Geometry check sheet. Reference: the model listing, model coordinates, mm. A direction names the side the tool comes from. Coordinates: 2 decimals unless noted, no trailing zeros. Order: outer loops, then holes, each group sorted by start corner. A loop starts at its lowest first (then second) coordinate and runs counter-clockwise, first axis right, second up. Notation, with made-up numbers: M 11.25,49.5 L 31.25,49.5 A20 cw 31.25,80.5 Z; hole C -34.75,44 d3. An arc over 180 degrees is marked long. Use CSV: the item, a comma, the result in double quotes. Start each with the question number.
```python
from build123d import *

# Parameters (mm, degrees)
SKETCH_2_W          = 170
SKETCH_2_H          = 20
EXTRUDE_1_DEPTH     = 23
CUT_EXTRUDE_1_DEPTH = 173.710740836
SKETCH_4_W          = 17
SKETCH_4_H          = 13
CUT_EXTRUDE_2_DEPTH = 30
CUT_EXTRUDE_3_DEPTH = 173.710740836
SKETCH_6_W          = 17.5
SKETCH_6_H          = 14.5
CUT_EXTRUDE_4_DEPTH = 173.710740836
SKETCH_7_W          = 27
SKETCH_7_H          = 23
SKETCH_7_R          = 1.25
EXTRUDE_2_DEPTH     = 3
CUT_EXTRUDE_START   = -3
SKETCH_7_3_R        = 2
CUT_EXTRUDE_5_DEPTH = 1.5


with BuildPart() as part:
    # 草图2 → 凸台-拉伸1 (new body)
    with BuildSketch(Plane(origin=(0, 0, 0), x_dir=(1, 0, 0), z_dir=(0, 1, 0))):
        with Locations((85, -10)):
            Rectangle(SKETCH_2_W, SKETCH_2_H)
    extrude(amount=EXTRUDE_1_DEPTH)

    # 草图3 → 切除-拉伸1 (cut, through all)
    with BuildSketch(Plane(origin=(0, 23, 0), x_dir=(1, 0, 0), z_dir=(0, 1, 0))):
        with BuildLine():
            ThreePointArc((161.6, -10), (159.341699476, -8.541699476), (158.941699476, -11.2))
            Line((158.941699476, -11.2), (161.058300524, -11.2))
            ThreePointArc((161.058300524, -11.2), (161.458300524, -10.658300524), (161.6, -10))
        make_face()
        with BuildLine():
            ThreePointArc((126.6, -10), (124.341699476, -8.541699476), (123.941699476, -11.2))
            Line((123.941699476, -11.2), (126.058300524, -11.2))
            ThreePointArc((126.058300524, -11.2), (126.458300524, -10.658300524), (126.6, -10))
        make_face()
    extrude(amount=-CUT_EXTRUDE_1_DEPTH, mode=Mode.SUBTRACT)

    # 草图4 → 切除-拉伸2 (cut)
    with BuildSketch(Plane(origin=(170, 0, 0), x_dir=(0, 0, -1), z_dir=(1, 0, 0))):
        with Locations((-8.5, 11.5)):
            Rectangle(SKETCH_4_W, SKETCH_4_H)
    extrude(amount=-CUT_EXTRUDE_2_DEPTH, mode=Mode.SUBTRACT)

    # 草图5 → 切除-拉伸3 (cut, through all)
    with BuildSketch(Plane(origin=(0, 23, 0), x_dir=(1, 0, 0), z_dir=(0, 1, 0))):
        with BuildLine():
            Line((117.5, -17), (117.5, -10))
            ThreePointArc((117.5, -10), (125, -2.5), (132.5, -10))
            Line((132.5, -10), (132.5, -17))
            Line((132.5, -17), (152.5, -17))
            Line((152.5, -17), (152.5, -10))
            ThreePointArc((152.5, -10), (160, -2.5), (167.5, -10))
            Line((167.5, -10), (167.5, -17))
            Line((167.5, -17), (170, -17))
            Line((170, -17), (170, 0))
            Line((170, 0), (0, 0))
            Line((0, 0), (0, -20))
            Line((0, -20), (102.5, -20))
            Line((102.5, -20), (102.5, -17))
            Line((102.5, -17), (117.5, -17))
        make_face()
    extrude(amount=-CUT_EXTRUDE_3_DEPTH, mode=Mode.SUBTRACT)

    # 草图6 → 切除-拉伸4 (cut, through all)
    with BuildSketch(Plane(origin=(0, 23, 0), x_dir=(1, 0, 0), z_dir=(0, 1, 0))):
        Polygon((152.5, -17), (102.5, -17), (102.5, -20), (170, -20), (170, -17), align=None)
        with Locations((161.25, -9.75)):
            Rectangle(SKETCH_6_W, SKETCH_6_H)
    extrude(amount=-CUT_EXTRUDE_4_DEPTH, mode=Mode.SUBTRACT)

    # 草图7 → 凸台-拉伸2 (add)
    with BuildSketch(Plane.XY.offset(17)):
        with Locations((125, 11.5)):
            Rectangle(SKETCH_7_W, SKETCH_7_H)
        with Locations((114.5, 19)):
            Circle(SKETCH_7_R, mode=Mode.SUBTRACT)
        with Locations((114.5, 4)):
            Circle(SKETCH_7_R, mode=Mode.SUBTRACT)
        with Locations((135.5, 4)):
            Circle(SKETCH_7_R, mode=Mode.SUBTRACT)
        with Locations((135.5, 19)):
            Circle(SKETCH_7_R, mode=Mode.SUBTRACT)
    extrude(amount=-EXTRUDE_2_DEPTH)

    # 草图7<3> → 切除-拉伸5 (cut)
    with BuildSketch(Plane.XY.offset(17).offset(CUT_EXTRUDE_START)):
        with Locations(Location((114.5, 19, 0), (0, 0, 180))):
            Circle(SKETCH_7_3_R)
        with Locations(Location((114.5, 4, 0), (0, 0, 180))):
            Circle(SKETCH_7_3_R)
        with Locations(Location((135.5, 4, 0), (0, 0, 180))):
            Circle(SKETCH_7_3_R)
        with Locations(Location((135.5, 19, 0), (0, 0, 180))):
            Circle(SKETCH_7_3_R)
    extrude(amount=CUT_EXTRUDE_5_DEPTH, mode=Mode.SUBTRACT)


solid = part.part
```
1) Gauge pin test, flat ends, axial feed: P1, Ø4, axis at y = 2.5, z = 10.5, coming from the +X side; P2, Ø3, axis at y = 17, z = 7, coming from the +X side; P3, Ø1.2, axis at y = 11, z = 12, coming from the -X side. Record the tip position at first contact, or that the pin passes through.
2) Section check A-A on x = 135.5. Record the boundary of the cut face in (y, z), then the cut area to 3 significant figures.
3) Set-up check for faces 5 (the face through (125, 12, 17)), 6 (the face through (113, 4, 15.5)), 7 (the face through (135, 12, 14)), 8 (the face through (125, 12, 11.2)), 9 (the face through (124.8, 0, 11.5)): record each of +Z, -Z, +X, -X, +Y, -Y from which the full face is reachable in a straight line by a thin tool's end or side.
4) Material ranges on line 1 along X through (y, z) = (19, 14.45); line 2 along Y through (x, z) = (114.5, 14.6); line 3 along X through (y, z) = (8.5, 10), recorded low to high.
5) Section check D-D on z = 10.5. Record the boundary of the cut face in (x, y).
6) Draft check along Y on faces 1 (the face through (117.5, 12, 12)), 2 (the face through (115.655, 3.521, 16.26)), 3 (the face through (116.498, 18.912, 14.74)), 4 (the face through (124.8, 23, 11.5)). Enter one of: +Y half, -Y half, draft (parallel to the pull), parting line (faces both ways), or undercut.
7) Section check B-B on y = 19. Record the boundary of the cut face in (x, z), then the cut area to 3 significant figures.
8) Section check C-C on x = 125. Record the boundary of the cut face in (y, z).
Results are:
1,P1,"stops at x = 132.5"
1,P2,"stops at x = 132.35"
1,P3,"stops at x = 117.5"
2,outline,"M 0,14 L 2,14 L 2,15.5 L 2.75,15.5 L 2.75,17 L 0,17 Z; M 5.25,15.5 L 6,15.5 L 6,14 L 17,14 L 17,15.5 L 17.75,15.5 L 17.75,17 L 5.25,17 Z; M 20.25,15.5 L 21,15.5 L 21,14 L 23,14 L 23,17 L 20.25,17 Z"
2,area,"49.5 mm²"
3,face 5,"+Z, +X, -X, +Y, -Y"
3,face 6,"-Z"
3,face 7,"-Z, +X, +Y, -Y"
3,face 8,"+Y, -Y"
3,face 9,"+Z, -Z, +X, -X, -Y"
4,line 1,"x = 111.5 to 112.5, 116.5 to 133.5, 137.5 to 138.5"
4,line 2,"y = 0 to 2, 6 to 17, 21 to 23"
4,line 3,"x = 117.5 to 123.4, 126.6 to 132.5"
5,outline,"M 117.5,0 L 123.48,0 L 123.48,23 L 117.5,23 Z; M 126.52,0 L 132.5,0 L 132.5,23 L 126.52,23 Z"
6,face 1,"draft"
6,face 2,"undercut"
6,face 3,"undercut"
6,face 4,"+Y half"
7,outline,"M 111.5,14 L 112.5,14 L 112.5,15.5 L 113.25,15.5 L 113.25,17 L 111.5,17 Z; M 115.75,15.5 L 116.5,15.5 L 116.5,14 L 117.5,14 L 117.5,10 A7.5 ccw 132.5,10 L 132.5,14 L 133.5,14 L 133.5,15.5 L 134.25,15.5 L 134.25,17 L 115.75,17 Z; M 136.75,15.5 L 137.5,15.5 L 137.5,14 L 138.5,14 L 138.5,17 L 136.75,17 Z; hole M 123.94,11.2 A1.6 ccw long 126.06,11.2 Z"
7,area,"202 mm²"
8,outline,"M 0,2.5 L 23,2.5 L 23,8.4 L 0,8.4 Z; M 0,11.2 L 23,11.2 L 23,17 L 0,17 Z"
